```python
from build123d import *

# Parameters (mm, degrees)
ESBO_O1_W                = 101.6
ESBO_O1_H                = 100
RESSALTO_EXTRUS_O1_DEPTH = 9.53
ESBO_O2_R                = 2.6
CORTE_EXTRUS_O1_DEPTH    = 20
ESBO_O3_R                = 32.51
CORTE_EXTRUS_O2_DEPTH    = 5
CORTE_EXTRUS_O3_REACH    = 73.454
ESBO_O4_R                = 27.5
CORTE_EXTRUS_O4_REACH    = 73.913
ESBO_O5_W                = 33.3
ESBO_O5_H                = 13
CORTE_EXTRUS_O5_REACH    = 73.913
ESBO_O6_W                = 6
ESBO_O6_H                = 29.667415493
CORTE_EXTRUS_O6_REACH    = 87.18
ESBO_O7_R                = 2.5


with BuildPart() as part:
    # Esboço1 → Ressalto-extrusão1 (new body)
    with BuildSketch(Plane(origin=(0, 0, 0), x_dir=(1, 0, 0), z_dir=(0, 1, 0))):
        Rectangle(ESBO_O1_W, ESBO_O1_H)
    extrude(amount=RESSALTO_EXTRUS_O1_DEPTH)

    # Esboço2 → Corte-extrusão1 (cut)
    with BuildSketch(Plane(origin=(0, 0, -50), x_dir=(-1, 0, 0), z_dir=(0, 0, -1))):
        with Locations((-45.8, 4.76)):
            Circle(ESBO_O2_R)
        with Locations((-22.8, 4.76)):
            Circle(ESBO_O2_R)
        with Locations((22.8, 4.76)):
            Circle(ESBO_O2_R)
        with Locations((45.8, 4.76)):
            Circle(ESBO_O2_R)
    extrude(amount=-CORTE_EXTRUS_O1_DEPTH, mode=Mode.SUBTRACT)

    # Esboço3 → Corte-extrusão2 (cut)
    with BuildSketch(Plane(origin=(0, 9.53, 0), x_dir=(1, 0, 0), z_dir=(0, 1, 0))):
        with Locations(Location((0, 0, 0), (0, 0, 270))):
            Circle(ESBO_O3_R)
    extrude(amount=-CORTE_EXTRUS_O2_DEPTH, mode=Mode.SUBTRACT)

    # Esboço4 → Corte-extrusão3 (cut, up to next)
    with BuildSketch(Plane(origin=(0, 4.53, 0), x_dir=(1, 0, 0), z_dir=(0, 1, 0)), mode=Mode.PRIVATE) as corte_extrus_o3_sk1:
        with Locations(Location((0, 0, 0), (0, 0, 270))):
            Circle(ESBO_O4_R)
    corte_extrus_o3_tool1 = extrude(corte_extrus_o3_sk1.sketch, amount=-CORTE_EXTRUS_O3_REACH, mode=Mode.PRIVATE) & part.part
    add(corte_extrus_o3_tool1.solids().sort_by_distance((0, 4.53, 0))[0], mode=Mode.SUBTRACT)

    # Esboço5 → Corte-extrusão4 (cut, up to next)
    with BuildSketch(Plane(origin=(0, 9.53, 0), x_dir=(1, 0, 0), z_dir=(0, 1, 0)), mode=Mode.PRIVATE) as corte_extrus_o4_sk1:
        with Locations((34.15, -43.5)):
            Rectangle(ESBO_O5_W, ESBO_O5_H)
    corte_extrus_o4_tool1 = extrude(corte_extrus_o4_sk1.sketch, amount=-CORTE_EXTRUS_O4_REACH, mode=Mode.PRIVATE) & part.part
    # Esboço5 → Corte-extrusão4 (cut, up to next)
    with BuildSketch(Plane(origin=(0, 9.53, 0), x_dir=(1, 0, 0), z_dir=(0, 1, 0)), mode=Mode.PRIVATE) as corte_extrus_o4_sk2:
        with Locations((-34.15, -43.5)):
            Rectangle(ESBO_O5_W, ESBO_O5_H)
    corte_extrus_o4_tool2 = extrude(corte_extrus_o4_sk2.sketch, amount=-CORTE_EXTRUS_O4_REACH, mode=Mode.PRIVATE) & part.part
    add(corte_extrus_o4_tool1.solids().sort_by_distance((34.15, 9.53, 43.5))[0], mode=Mode.SUBTRACT)
    add(corte_extrus_o4_tool2.solids().sort_by_distance((-34.15, 9.53, 43.5))[0], mode=Mode.SUBTRACT)

    # Esboço6 → Corte-extrusão5 (cut, up to next)
    with BuildSketch(Plane(origin=(0, 9.53, 0), x_dir=(1, 0, 0), z_dir=(0, 1, 0)), mode=Mode.PRIVATE) as corte_extrus_o5_sk1:
        with Locations((0, -35.166292254)):
            Rectangle(ESBO_O6_W, ESBO_O6_H)
    corte_extrus_o5_tool1 = extrude(corte_extrus_o5_sk1.sketch, amount=-CORTE_EXTRUS_O5_REACH, mode=Mode.PRIVATE) & part.part
    add(corte_extrus_o5_tool1.solids().sort_by_distance((0, 9.53, 35.166292))[0], mode=Mode.SUBTRACT)

    # Corte-extrusão6: up to this face of the body (flat: up to its plane)
    corte_extrus_o6_end = Plane(part.part.faces().sort_by_distance((17.5, 4.765, 43.5))[0])
    # Esboço7 → Corte-extrusão6 (cut, up to the picked face)
    with BuildSketch(Plane.ZY.offset(17.5), mode=Mode.PRIVATE) as corte_extrus_o6_sk1:
        with Locations((45, 4.765)):
            Circle(ESBO_O7_R)
    corte_extrus_o6_tool1 = split(extrude(corte_extrus_o6_sk1.sketch, amount=-CORTE_EXTRUS_O6_REACH, mode=Mode.PRIVATE), bisect_by=corte_extrus_o6_end, keep=Keep.BOTH, mode=Mode.PRIVATE)
    add(corte_extrus_o6_tool1.solids().sort_by(Axis((-17.5, 4.765, 45), (1, 0, 0)))[0], mode=Mode.SUBTRACT)


solid = part.part
```
Could you check a few things on this model? Use its own coordinates, in mm. A direction names the side the tool comes from. Give positions to 0.01 mm unless a question says otherwise; leave off trailing zeros. Loops run counter-clockwise (first coordinate to the right, second up) from the corner with the lowest first, then second, coordinate; pieces in that order, holes last. Notation, with made-up numbers: (31, 65) - (42, 65) arc R32 ccw to (42, 104) - close; hole circle Ø11 at (34, 88.5). An arc over 180 degrees is marked (long way). Answer in a Markdown table with one row per item. Add a question column.
Q1. If we section it at A-A (z = 45): List the corners of the cut face in (x, y) for me (3 decimals).
Q2. If we section it at D-D (z = -8): List the corners of the cut face in (x, y) for me.
Q3. For pin 1 (1.6 mm diameter, centred on x = -22, y = 6, fed in from -Z); pin 2 (4.5 mm diameter, centred on x = 45.8, y = 4.76, fed in from +Z); pin 3 (5 mm diameter, centred on y = 3, z = 42, fed in from -X), each with a flat end and sliding along its axis, tell me the tip position at first contact or that it passes through.
Q4. We'd pull the mould along Y, two halves only. Please class faces 1 (the face through (23, 5, -30)), 2 (the face through (-3, 5, 39)), 3 (the face through (7, 4.53, -27)), 4 (the face through (48.397, 4.874, -40.14)): +Y half, -Y half, draft (parallel to the pull), parting line (faces both ways), or undercut.
Q5. If we section it at C-C (x = 22.8): List the corners of the cut face in (y, z) for me.
Q6. Please list where these lines run through material, in increasing order: L1, parallel to X at y = 4.5, z = 37.5; L2, parallel to X at y = 2.9, z = 0; L3, parallel to Z at x = -5, y = 3.5. Write a range as from..to.
Q7. If we section it at B-B (x = -4.5): List the corners of the cut face in (y, z) for me (3 decimals).
Q8. Which directions (+Z, -Z, +X, -X, +Y, -Y) give clear straight access to the entire face, cutting with the end or side of a thin tool? Please do faces 5 (the face through (1.39, 7.06, -32.48)), 6 (the face through (-48.28, 5.54, -40.14)), 7 (the face through (-34, 5, 37)).
The answers:
| question | item | result |
|---|---|---|
| 1 | outline | (-17.5, 0) - (-3, 0) - (-3, 2.265) - (-17.5, 2.265) - close; (-17.5, 7.265) - (-3, 7.265) - (-3, 9.53) - (-17.5, 9.53) - close; (3, 0) - (17.5, 0) - (17.5, 2.265) - (3, 2.265) - close; (3, 7.265) - (17.5, 7.265) - (17.5, 9.53) - (3, 9.53) - close |
| 2 | outline | (-50.8, 0) - (-26.31, 0) - (-26.31, 4.53) - (-31.51, 4.53) - (-31.51, 9.53) - (-50.8, 9.53) - close; (26.31, 0) - (50.8, 0) - (50.8, 9.53) - (31.51, 9.53) - (31.51, 4.53) - (26.31, 4.53) - close |
| 3 | pin 1 | stops at z = -30 |
| 3 | pin 2 | stops at z = 37 |
| 3 | pin 3 | stops at x = -17.5 |
| 4 | face 1 | undercut |
| 4 | face 2 | draft |
| 4 | face 3 | +Y half |
| 4 | face 4 | undercut |
| 5 | outline | (0, -50) - (2.16, -50) - (2.16, -30) - (7.36, -30) - (7.36, -50) - (9.53, -50) - (9.53, -23.17) - (4.53, -23.17) - (4.53, -15.38) - (0, -15.38) - close; (0, 15.38) - (4.53, 15.38) - (4.53, 23.17) - (9.53, 23.17) - (9.53, 37) - (0, 37) - close |
| 6 | L1 | x = -17.5..-3, 3..17.5 |
| 6 | L2 | x = -50.8..-27.5, 27.5..50.8 |
| 6 | L3 | z = -50..-27.04, 27.04..42.84, 47.16..50 |
| 7 | outline | (0, -50) - (9.53, -50) - (9.53, -32.197) - (4.53, -32.197) - (4.53, -27.129) - (0, -27.129) - close; (0, 27.129) - (4.53, 27.129) - (4.53, 32.197) - (9.53, 32.197) - (9.53, 50) - (0, 50) - close; hole circle Ø5 at (4.765, 45) |
| 8 | face 5 | +Y |
| 8 | face 6 | -Z |
| 8 | face 7 | +Z, -X, +Y, -Y |
